from build123d import *

# Parameters (mm, degrees)
EXTRUDE_1_DEPTH = 200
FILLET_1_R      = 3
FILLET_2_R      = 5
CHAMFER_1_SIZE  = 7
CHAMFER_1_SIZE2 = 7.807485502
CHAMFER_2_SIZE  = 2
CHAMFER_3_SIZE  = 0.4


with BuildPart() as part:
    # 草图1 → 凸台-拉伸1 (new body)
    with BuildSketch(Plane(origin=(0, 0, 0), x_dir=(1, 0, 0), z_dir=(0, 1, 0))):
        Polygon((0, 0), (0, 30), (-30, 0), (-20, 0), (-20, -3), (-37.242640687, -3), (3, 37.242640687), (3, -3), (-8, -3), (-8, 0), align=None)
    extrude(amount=EXTRUDE_1_DEPTH)

    # 圆角1
    fillet_1_edges = [part.edges().sort_by_distance(p)[0] for p in [
        (0, 100, 0),
        (0, 100, -30),
        (-30, 100, 0),
    ]]
    fillet(fillet_1_edges, radius=FILLET_1_R)

    # 圆角2
    fillet_2_edges = [part.edges().sort_by_distance(p)[0] for p in [
        (3, 100, -37.242640687),
    ]]
    fillet(fillet_2_edges, radius=FILLET_2_R)

    # 倒角1
    chamfer_1_edges = [part.edges().sort_by_distance(p)[0] for p in [
        (-37.242640687, 100, 3),
    ]]
    chamfer_1_side = [part.faces().sort_by_distance(p)[0] for p in [
        (-21.389087297, 100, -12.853553391),
    ]]
    chamfer(chamfer_1_edges, length=CHAMFER_1_SIZE, length2=CHAMFER_1_SIZE2, reference=chamfer_1_side[0])

    # 倒角2
    chamfer_2_edges = [part.edges().sort_by_distance(p)[0] for p in [
        (3, 100, 3),
    ]]
    chamfer(chamfer_2_edges, length=CHAMFER_2_SIZE)

    # 倒角3
    chamfer_3_edges = [part.edges().sort_by_distance(p)[0] for p in [
        (-3.5, 200, 3),
        (-3.5, 0, 3),
        (-20, 100, 3),
        (-8, 100, 3),
        (-24.717577593, 0, 3),
        (-24.717577593, 200, 3),
    ]]
    chamfer(chamfer_3_edges, length=CHAMFER_3_SIZE)


solid = part.part
Model file for the job. Use its own axes, mm. A direction names the side the tool comes from. Give positions to 0.01 mm unless a question says otherwise; leave off trailing zeros. Order: outer loops, then holes, each group sorted by start corner. A loop starts at its lowest first (then second) coordinate and runs counter-clockwise, first axis right, second up. Notation, with made-up numbers: (10.5, -38) -> (29.5, -38) arc R9 ccw to (29.5, -30) -> close; hole circle Ø3 at (-16, 49). An arc over 180 degrees is marked (long way). Use CSV: the item, a comma, the result in double quotes.
1. Band-saw the part on C-C, the plane x = -12. Give the cut face in (y, z).
Outcome:
outline,"(0, -22.24) -> (200, -22.24) -> (200, -18) -> (0, -18) -> close"
2. Band-saw the part on B-B, the plane z = -10. Give the cut face in (x, y).
Outcome:
outline,"(-24.24, 0) -> (-20, 0) -> (-20, 200) -> (-24.24, 200) -> close; (0, 0) -> (3, 0) -> (3, 200) -> (0, 200) -> close"
3. Drop flat-ended pins along their axis: pin 1 (16 mm diameter, centred on y = 78, z = -8, fed in from -X); pin 2 (3 mm diameter, centred on y = 149.5, z = 1, fed in from -X); pin 3 (3 mm diameter, centred on y = 167.5, z = -5, fed in from -X); pin 4 (4 mm diameter, centred on x = -13, z = -12, fed in from +Y). Give the stop position or say it passes through.
Outcome:
pin 1,"x = -32.29"
pin 2,"x = -31.46"
pin 3,"x = -30.74"
pin 4,"through"
4. Drill centre lines: line 1 along X through (y, z) = (119, -2); line 2 along X through (y, z) = (178, -0.5); line 3 along Z through (x, y) = (-23, 121). Where is each one in solid material? Low to high. Write a range as from..to.
Outcome:
line 1,"-32.24..-25.59, -0.17..3"
line 2,"-31.46..-24.42, -1.34..3"
line 3,"-11.24..-7, -0.01..3"
5. 3-axis set-ups, long thin cutter, end or side, ignore diameter. For faces 1 (the flat face through (-3, 99, 3)), 2 (the flat face through (0, 99, -13)): which of +Z, -Z, +X, -X, +Y, -Y reach the whole face in a straight line?
Outcome:
face 1,"+Z, +X, -X, +Y, -Y"
face 2,"+Y, -Y"
6. Band-saw the part on A-A, the plane y = 21.5. Give the cut face in (x, z).
Outcome:
outline,"(-32.29, -1.95) -> (-5.54, -28.71) arc R5 ccw to (3, -25.17) -> (3, 1) -> (1, 3) -> (-7.6, 3) -> (-8, 2.6) -> (-8, 0) -> (-3, 0) arc R3 cw to (0, -3) -> (0, -22.76) arc R3 cw to (-5.12, -24.88) -> (-24.88, -5.12) arc R3 cw to (-22.76, 0) -> (-20, 0) -> (-20, 2.6) -> (-20.4, 3) -> (-29.44, 3) -> close"
7. Mould opens along X. For faces 3 (the flat face through (-13, 0, -18)), 4 (the cylindrical face through (-0.01, 101.4, -29.76)), 5 (the flat face through (-6, 99, 0)) say: +X half, -X half, draft (parallel to the pull), parting line (faces both ways), or undercut.
Outcome:
face 3,"draft"
face 4,"parting line"
face 5,"undercut"
